from build123d import *

# Parameters (mm, degrees)
F0_R     = 3
F1_DEPTH = 5
F2_R     = 3
F3_DEPTH = 4
F5_D     = 3
F5_DEPTH = 15


with BuildPart() as f1:
    # F0 (on Top) → F1 (new body)
    with BuildSketch(Plane.XY):
        Circle(F0_R)
    extrude(amount=-F1_DEPTH)

    # F2 (on Top) → F3 (join)
    with BuildSketch(Plane.XY):
        Circle(F2_R)
    extrude(amount=F3_DEPTH)

    # F5
    with Locations(Plane.XY.offset(4)):
        with Locations((0, 0)):
            Hole(F5_D / 2, depth=F5_DEPTH)


solid = f1.part
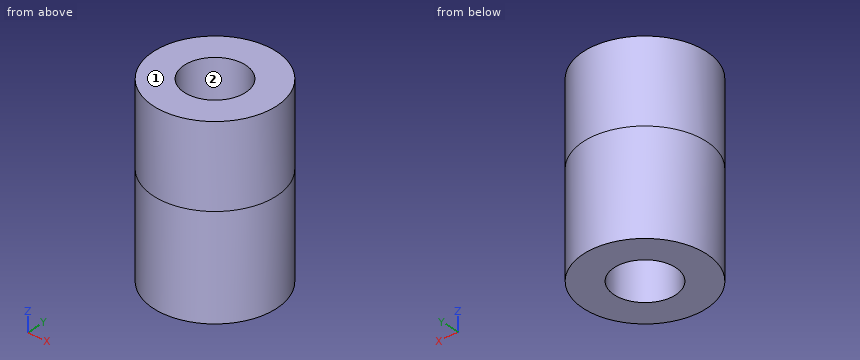
The model under review builds one solid part; all positions refer to its coordinate system, in mm. Face numbers are marked on the shaded views. Round coordinates to 2 decimals unless told otherwise and drop trailing zeros. Loops run counter-clockwise (first coordinate to the right, second up) from the corner with the lowest first, then second, coordinate; pieces in that order, holes last. Notation, with made-up numbers: M -26.75,16.25 L 0.25,16.25 A17 cw 0.25,41.25 Z; hole C -27,56.25 d4. An arc over 180 degrees is marked long. Answer as a JSON object with one key per item and string values.
Item 1: The part is to be moulded in two halves that separate along X. For the marked faces 1 and 2, say which applies: +X half, -X half, draft (parallel to the pull), parting line (faces both ways), or undercut.
Check sheet entries:
{"face 1": "draft", "face 2": "undercut"}
Item 2: Clearance check with flat-ended pins moving along their axes: P1, Ø2.5, axis at x = 0, y = 0, coming from the +Z side; P2, Ø1.5, axis at x = 1, z = 3, coming from the +Y side. State where each tip first meets the part, or that it passes through.
Check sheet entries:
{"P1": "through", "P2": "y = 2.99"}
Item 3: We need section D-D, the plane y = -2.25. State the section outline as (x, z) points, and give its area (3 significant figures).
Check sheet entries:
{"outline": "M -1.98,-5 L 1.98,-5 L 1.98,4 L -1.98,4 Z", "area": "35.7 mm2"}
Item 4: For line 1 along Y through (x, z) = (0, 1); line 2 along Y through (x, z) = (1.25, 3.5); line 3 along X through (y, z) = (-0.7, 2.75), list the stretches that pass through material, from the lowest coordinate up.
Check sheet entries:
{"line 1": "-3 to -1.5, 1.5 to 3", "line 2": "-2.73 to -0.83, 0.83 to 2.73", "line 3": "-2.92 to -1.33, 1.33 to 2.92"}
Item 5: We need section C-C, the plane z = 3. State the section outline as (x, y) points, and give its area (3 significant figures).
Check sheet entries:
{"outline": "C 0,0 d6; hole C 0,0 d3", "area": "21.2 mm2"}
Item 6: We need section A-A, the plane x = 0. State the section outline as (y, z) points, and give its area (3 significant figures).
Check sheet entries:
{"outline": "M -3,-5 L -1.5,-5 L -1.5,4 L -3,4 Z; M 1.5,-5 L 3,-5 L 3,4 L 1.5,4 Z", "area": "27.0 mm2"}
